Part print with two shaded views. Sizes in mm from the minimum x, y, z corner. A direction names the side the tool comes from. Round coordinates to 2 decimals unless told otherwise and drop trailing zeros. Order: outer loops, then holes, each group sorted by start corner. A loop starts at its lowest first (then second) coordinate and runs counter-clockwise, first axis right, second up. Notation, with made-up numbers: M -7.5,-37 L 44.5,-37 A27 cw 44.5,-7 Z; hole C 82,-14.5 d10. An arc over 180 degrees is marked long. Return JSON: item names as keys, results as strings. Group by question number.
Item 1: Probe line 1 along X through (y, z) = (9.5, 17.5) (1 decimal); line 2 along Z through (x, y) = (5.5, 3.5); line 3 along X through (y, z) = (5.75, 29). List the from-to ranges inside material, lowest first.
Item 2: Slice it at A-A on z = 11.5. Write the cut outline in (x, y) (1 decimal).
Item 3: Pin check, flat tips, straight feed: pin 1 Ø3 at (x, z) = (13.5, 32.5) entering from -Y; pin 2 Ø1 at (y, z) = (12, 18) entering from +X (1 decimal); pin 3 Ø2 at (x, z) = (11, 29.5) entering from -Y. Stop position of each tip, or through.
Item 4: Which spindle directions (+Z, -Z, +X, -X, +Y, -Y) get a long thin tool onto all of the face, cutting with end or side? Do the marked faces 1 and 2. Say none if no direction does.
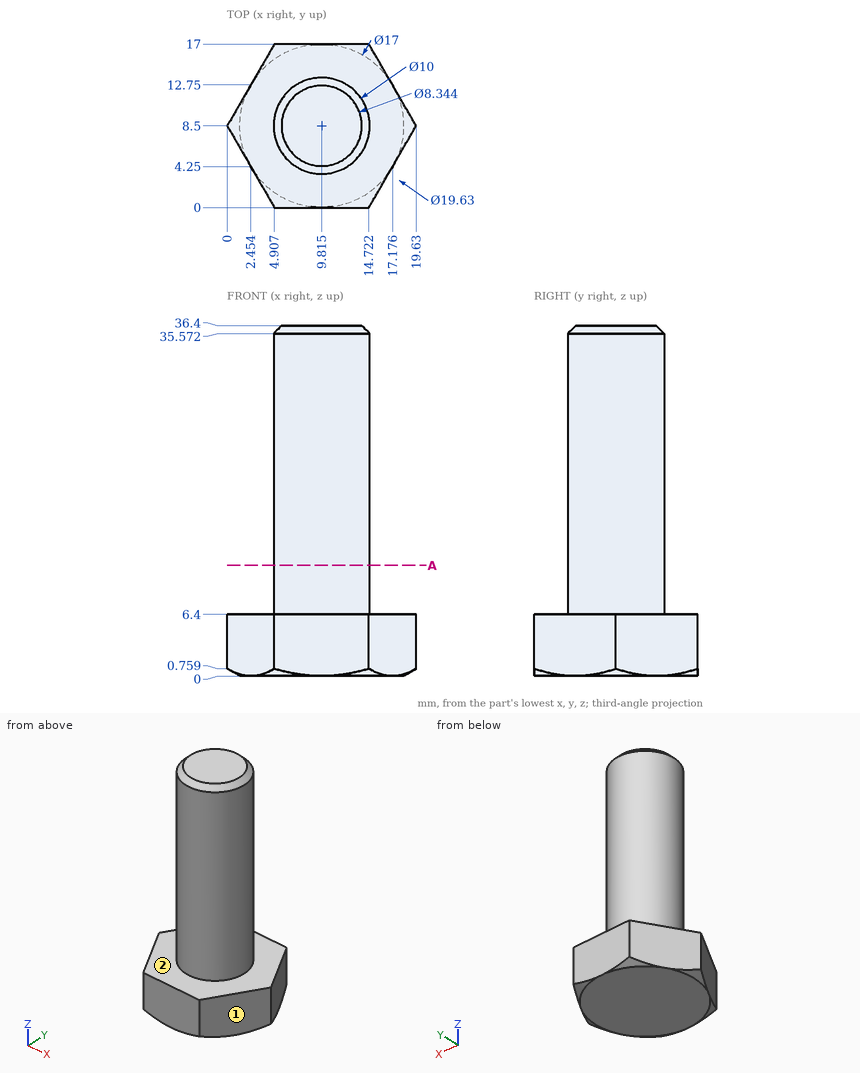
Output values:
{
 "1": {"line 1": "4.9 to 14.7", "line 2": "0 to 6.4", "line 3": "5.64 to 13.99"},
 "2": {"outline": "C 9.8,8.5 d10"},
 "3": {"pin 1": "y = 4", "pin 2": "x = 13.8", "pin 3": "y = 3.5"},
 "4": {"face 1": "+Z, -Z, +X, -Y", "face 2": "+Z"}
}
